Verification items for the finished model (mm, model axes). A direction names the side the tool comes from. Round coordinates to 2 decimals unless told otherwise and drop trailing zeros. Write each loop counter-clockwise with the first axis right and the second up, starting at its lowest first coordinate (ties: lowest second). Pieces come first, ordered by that corner, then holes. Notation, with made-up numbers: M -12,15 L 38,15 A24 ccw 38,52 Z; hole C -26.75,-16 d10. An arc over 180 degrees is marked long. One line per item, written item: value. Start each with the question number.
Item 1: Tool access check on faces 5 (the face through (-17.974, -17.912, 50.465)), 6 (the face through (17.912, -17.974, 50.465)), 7 (the face through (8.4, 9.97, 68.21)), 8 (the face through (-17.912, 17.974, 50.465)), 9 (the face through (0, 20.15, 50)). Record the directions out of +Z, -Z, +X, -X, +Y, -Y that give a thin tool (end or side, any length) a straight path to the whole face; none if there is none.
Item 2: Gauge pin test, flat ends, axial feed: pin 1 (1.5 mm diameter, centred on x = -3, z = 51, fed in from +Y); pin 2 (2.5 mm diameter, centred on y = 7, z = 50, fed in from -X); pin 3 (2 mm diameter, centred on x = 2.5, z = 63, fed in from +Y). Record the tip position at first contact, or that the pin passes through.
Item 3: Draft check along Y on faces 1 (the face through (21.15, 0, 24)), 2 (the face through (-8.4, -9.97, 68.21)), 3 (the face through (10, 10, 53)), 4 (the face through (-2.38, -10.74, 83.99)). Enter one of: +Y half, -Y half, draft (parallel to the pull), parting line (faces both ways), or undercut.
Item 4: Section check C-C, the plane z = 64.5. Record the cut outline in (x, y).
Item 5: Section check A-A, the plane y = 0. Record the cut outline in (x, z).
Item 6: Thickness scan on probe 1 along Z at (x, y) = (15, 15.5); probe 2 along Y at (x, z) = (13, 52). Record the ranges inside material, lowest first. Write a range as from..to.
from build123d import *

# Parameters (mm, degrees)
SCHIZZO1_W                   = 42.3
SCHIZZO1_H                   = 42.3
ESTRUSIONE_ESTRUSIONE1_DEPTH = 48
SMUSSO1_SIZE                 = 5
ESTRUSIONE_ESTRUSIONE2_DEPTH = 5
SCHIZZO3_R                   = 18
ESTRUSIONE_ESTRUSIONE3_DEPTH = 30
SCHIZZO4_R                   = 11
ESTRUSIONE_ESTRUSIONE4_DEPTH = 2
SCHIZZO7_R                   = 1.5
TAGLIO_ESTRUSIONE2_DEPTH     = 30
RIPETIZIONECIRCOLARE1_COUNT  = 4


with BuildPart() as part:
    # Schizzo1 → Estrusione-Estrusione1 (new body)
    with BuildSketch(Plane.XY):
        Rectangle(SCHIZZO1_W, SCHIZZO1_H)
    extrude(amount=ESTRUSIONE_ESTRUSIONE1_DEPTH)

    # Smusso1
    smusso1_edges = [part.edges().sort_by_distance(p)[0] for p in [
        (-21.15, 21.15, 24),
        (21.15, 21.15, 24),
        (21.15, -21.15, 24),
        (-21.15, -21.15, 24),
    ]]
    chamfer(smusso1_edges, length=SMUSSO1_SIZE)

    # Schizzo2 → Estrusione-Estrusione2 (add)
    with BuildSketch(Plane.XY.offset(48)):
        Polygon((-20.15, 15.735786438), (-20.15, -15.735786438), (-15.735786438, -20.15), (15.735786438, -20.15), (20.15, -15.735786438), (20.15, 15.735786438), (15.735786438, 20.15), (-15.735786438, 20.15), align=None)
    extrude(amount=ESTRUSIONE_ESTRUSIONE2_DEPTH)

    # Schizzo3 → Estrusione-Estrusione3 (add)
    with BuildSketch(Plane.XY.offset(53)):
        Circle(SCHIZZO3_R)
    extrude(amount=ESTRUSIONE_ESTRUSIONE3_DEPTH)

    # Schizzo4 → Estrusione-Estrusione4 (add)
    with BuildSketch(Plane.XY.offset(83)):
        Circle(SCHIZZO4_R)
    extrude(amount=ESTRUSIONE_ESTRUSIONE4_DEPTH)

    # Schizzo7 → Taglio-Estrusione2 (cut)
    with BuildSketch(Plane.XY.offset(83)):
        with Locations((9.899494937, 9.899494937)):
            Circle(SCHIZZO7_R)
    taglio_estrusione2 = extrude(amount=-TAGLIO_ESTRUSIONE2_DEPTH, mode=Mode.SUBTRACT)

    # RipetizioneCircolare1: Taglio-Estrusione2 ×4 about axis
    ripetizionecircolare1_axis = Axis((0, 0, 0), (0, 0, 1))
    for i in range(1, RIPETIZIONECIRCOLARE1_COUNT):
        add(taglio_estrusione2.rotate(ripetizionecircolare1_axis, i * 360 / RIPETIZIONECIRCOLARE1_COUNT), mode=Mode.SUBTRACT)


solid = part.part
Response values:
1. face 5: +Z, -X, -Y
1. face 6: +Z, +X, -Y
1. face 7: +Z
1. face 8: +Z, -X, +Y
1. face 9: +Z, +X, -X, +Y
2. pin 1: stops at y = 20.15
2. pin 2: stops at x = -20.15
2. pin 3: stops at y = 17.94
3. face 1: draft
3. face 2: undercut
3. face 3: undercut
3. face 4: parting line
4. outline: C 0,0 d36; hole C -9.9,-9.9 d3; hole C -9.9,9.9 d3; hole C 9.9,-9.9 d3; hole C 9.9,9.9 d3
5. outline: M -21.15,0 L 21.15,0 L 21.15,48 L 20.15,48 L 20.15,53 L 18,53 L 18,83 L 11,83 L 11,85 L -11,85 L -11,83 L -18,83 L -18,53 L -20.15,53 L -20.15,48 L -21.15,48 Z
6. probe 1: z = 0..53
6. probe 2: y = -20.15..20.15
